Study the drawing (mm; zero at the part's minimum x, y, z) and answer. A direction names the side the tool comes from. Round coordinates to 2 decimals unless told otherwise and drop trailing zeros. Write each loop counter-clockwise with the first axis right and the second up, starting at its lowest first coordinate (ties: lowest second). Pieces come first, ordered by that corner, then holes.
(1) Find the intervals of material crossed by probe 1 along Z at (x, y) = (8.75, 11); probe 2 along Y at (x, z) = (7.5, 163.6); probe 3 along Z at (x, y) = (14.25, 6.25), in increasing order.
(2) Each of these flat-tipped pins is pushed along its axis until it touches: pin 1 Ø2.5 at (x, y) = (7.5, 10) entering from -Z; pin 2 Ø1.5 at (x, z) = (7.5, 38.5) entering from -Y; pin 3 Ø7.5 at (x, z) = (8.5, 142.5) entering from -Y. Where does it stop, or does it pass through?
(3) The mould has two halves that part along Z. Classify the marked faces 3, 4 and 5: +Z half, -Z half, draft (parallel to the pull), parting line (faces both ways), or undercut.
(4) A cutting plane is placed at A-A, the plane y = 23.5. Give the vertices of the cut face in (x, z).
(5) A cutting plane is placed at B-B, the plane x = 7.5. Give the vertices of the cut face in (y, z).
(6) For the marked faces 1 and 2, determine the directions among +Z, -Z, +X, -X, +Y, -Y from which every point of the face is accessible in a straight line to the end or side of a thin tool.
(7) A cutting plane is placed at D-D, the plane z = 110.5. Give the vertices of the cut face in (x, y), and give its area (3 significant figures).
(8) A cutting plane is placed at C-C, the plane y = 10. Give the vertices of the cut face in (x, z).
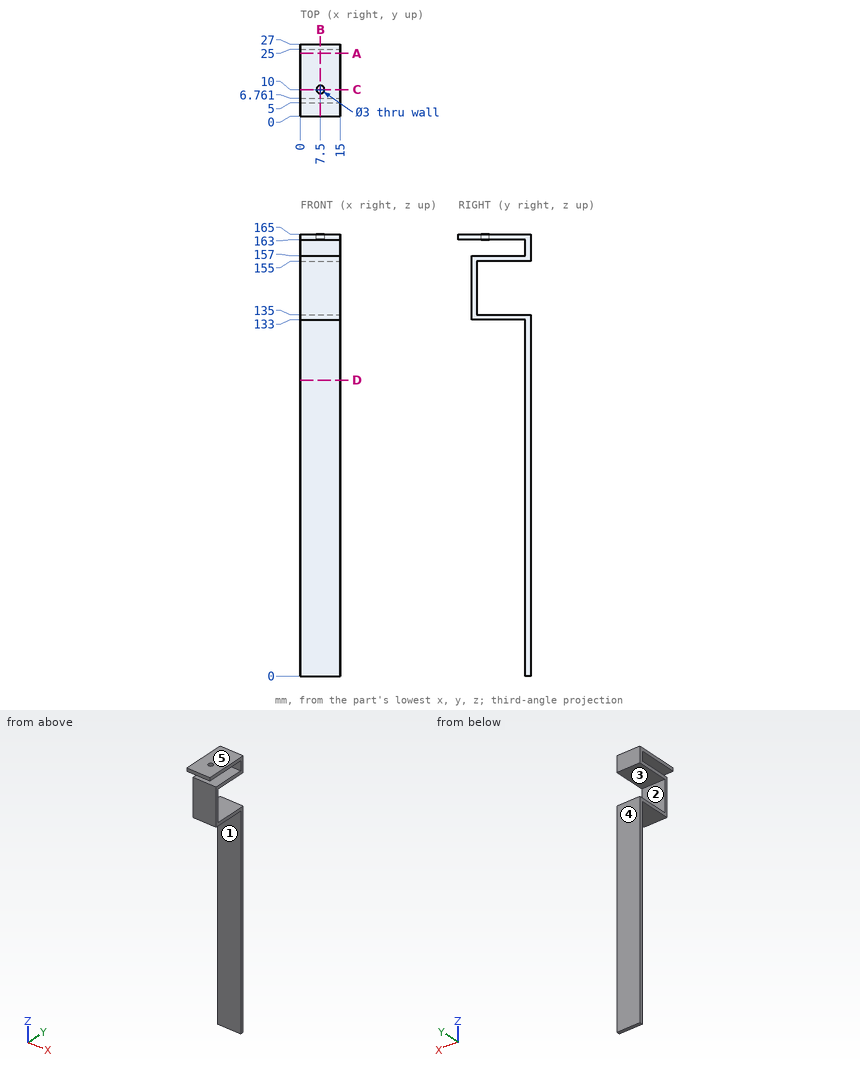
Solutions:
1. probe 1: z = 133 to 135, 155 to 157, 163 to 165
1. probe 2: y = 0 to 8.5, 11.5 to 27
1. probe 3: z = 133 to 157, 163 to 165
2. pin 1: stops at z = 133
2. pin 2: stops at y = 25
2. pin 3: stops at y = 5
3. face 3: undercut
3. face 4: draft
3. face 5: +Z half
4. outline: (0, 133) - (15, 133) - (15, 135) - (0, 135) - close; (0, 155) - (15, 155) - (15, 157) - (0, 157) - close; (0, 163) - (15, 163) - (15, 165) - (0, 165) - close
5. outline: (0, 163) - (8.5, 163) - (8.5, 165) - (0, 165) - close; (5, 133) - (25, 133) - (25, 0) - (27, 0) - (27, 135) - (6.76, 135) - (6.76, 155) - (27, 155) - (27, 165) - (11.5, 165) - (11.5, 163) - (25, 163) - (25, 157) - (5, 157) - close
6. face 1: -Z, +X, -X, -Y
6. face 2: +X, -X, +Y
7. outline: (0, 25) - (15, 25) - (15, 27) - (0, 27) - close
7. area: 30.0 mm2
8. outline: (0, 133) - (15, 133) - (15, 135) - (0, 135) - close; (0, 155) - (15, 155) - (15, 157) - (0, 157) - close; (0, 163) - (6, 163) - (6, 165) - (0, 165) - close; (9, 163) - (15, 163) - (15, 165) - (9, 165) - close
